```python
from build123d import *

# Parameters (mm, degrees)
SKETCH1_W           = 12.8
SKETCH1_H           = 5.8
BOSS_EXTRUDE1_DEPTH = 6.5
SKETCH2_R           = 1
CUT_EXTRUDE1_DEPTH  = 16.5
SKETCH3_W           = 0.9
SKETCH3_H           = 0.6
BOSS_EXTRUDE2_DEPTH = 3.5
BOSS_EXTRUDE3_DEPTH = 5.8
BOSS_EXTRUDE4_DEPTH = 2


with BuildPart() as part:
    # Sketch1 → Boss-Extrude1 (new body)
    with BuildSketch(Plane(origin=(0, 0, 0), x_dir=(1, 0, 0), z_dir=(0, 1, 0))):
        Rectangle(SKETCH1_W, SKETCH1_H)
    extrude(amount=BOSS_EXTRUDE1_DEPTH)

    # Sketch2 → Cut-Extrude1 (cut)
    with BuildSketch(Plane.XY.offset(2.9)):
        with Locations((-3.25, 1.4)):
            Circle(SKETCH2_R)
        with Locations((3.25, 1.4)):
            Circle(SKETCH2_R)
    extrude(amount=-CUT_EXTRUDE1_DEPTH, mode=Mode.SUBTRACT)

    # Sketch3 → Boss-Extrude2 (add)
    with BuildSketch(Plane.XZ):
        with Locations((-5.15, 0)):
            Rectangle(SKETCH3_W, SKETCH3_H)
        Rectangle(SKETCH3_W, SKETCH3_H)
        with Locations((5.15, 0)):
            Rectangle(SKETCH3_W, SKETCH3_H)
    extrude(amount=BOSS_EXTRUDE2_DEPTH)

    # Sketch4 → Boss-Extrude3 (add)
    with BuildSketch(Plane.XY.offset(2.9)):
        with BuildLine():
            Line((-3.1, 6.5), (-3.1, 7.3))
            ThreePointArc((-3.1, 7.3), (-2.1, 8.3), (-1.1, 7.3))
            Line((-1.1, 7.3), (-1.1, 6.5))
            Line((-1.1, 6.5), (-3.1, 6.5))
        make_face()
    extrude(amount=-BOSS_EXTRUDE3_DEPTH)

    # Sketch5 → Boss-Extrude4 (add, symmetric)
    with BuildSketch(Plane.XY):
        Polygon((-5.1, 6.5), (-5.1, 8.3), (8.241176471, 10.364705882), (8.294705882, 10.018823529), (-4.75, 8), (-4.75, 6.5), align=None)
    extrude(amount=BOSS_EXTRUDE4_DEPTH, both=True)


solid = part.part
```
Geometry: final body of the model. Coordinates: model frame, mm. A direction names the side the tool comes from. Give positions to 0.01 mm unless a question says otherwise; leave off trailing zeros. Order: outer loops, then holes, each group sorted by start corner. A loop starts at its lowest first (then second) coordinate and runs counter-clockwise, first axis right, second up. Notation, with made-up numbers: (32, 43) -> (76, 43) arc R12 cw to (76, 59) -> close; hole circle Ø2 at (21.5, -32). An arc over 180 degrees is marked (long way). Write each question's results on one line, items separated by ' | '. Start each with the question number.
1) Line query: line 1 (Y direction, x = -3.25, z = -0.05); line 2 (Y direction, x = 3.25, z = -0.85); line 3 (X direction, y = 0.75, z = 2.2). Output: solid intervals per line, ascending. Write a range as from..to.
2) Set-up query: faces 4 (the flat face through (5, -2, 0.3)), 5 (the flat face through (6.4, 3, 0)), 6 (the flat face through (0.6, 9, -2)), 7 (the flat face through (5, -2, -0.3)). Return all of +Z, -Z, +X, -X, +Y, -Y with unobstructed straight access to the full face (end or side cutting, diameter ignored); none if empty.
3) Draft query along X for faces 1 (the flat face through (0, -2, -0.3)), 2 (the cylindrical face through (-4.25, 1.44, 0.04)), 3 (the flat face through (-5.1, 7, 0)). Return one class per face: pulls with the +X half, pulls with the -X half, needs draft (parallel to the pull), parting line crosses it, or undercut.
4) Section C-C (x = 3.25). Return loops of the section in (y, z), then the cut area to 3 significant figures.
5) Section B-B (z = 1.05). Return loops of the section in (x, y).
6) First-contact query: pin 1 (3 mm diameter, centred on x = 2.5, z = -2, fed in from +Y); pin 2 (0.7 mm diameter, centred on x = 0, y = -2.5, fed in from -Z); pin 3 (0.9 mm diameter, centred on y = 7, z = 0, fed in from -X); pin 4 (1.6 mm diameter, centred on x = 3.25, y = 1.4, fed in from -Z). Flat tips, straight axial feed; report the tip coordinate or a pass-through.
7) Section D-D (y = 7.75). Return loops of the section in (x, z).
8) Section A-A (y = 1.4). Return loops of the section in (x, z), then the cut area to 3 significant figures.
Calculated:
1) line 1: 0..0.4, 2.4..6.5, 8.23..8.59 | line 2: 0..0.4, 2.4..6.5, 9.24..9.59 | line 3: -6.4..-4.01, -2.49..2.49, 4.01..6.4
2) face 4: +Z, +X, -X, -Y | face 5: +Z, -Z, +X, -Y | face 6: -Z, -X, +Y | face 7: -Z, +X, -X, -Y
3) face 1: needs draft | face 2: undercut | face 3: pulls with the -X half
4) outline: (0, -2.9) -> (0.4, -2.9) -> (0.4, 2.9) -> (0, 2.9) -> close; (2.4, -2.9) -> (6.5, -2.9) -> (6.5, 2.9) -> (2.4, 2.9) -> close; (9.24, -2) -> (9.59, -2) -> (9.59, 2) -> (9.24, 2) -> close | area: 27.5 mm2
5) outline: (-6.4, 0) -> (6.4, 0) -> (6.4, 6.5) -> (-1.1, 6.5) -> (-1.1, 7.3) arc R1 ccw to (-3.1, 7.3) -> (-3.1, 6.5) -> (-4.75, 6.5) -> (-4.75, 8) -> (8.29, 10.02) -> (8.24, 10.36) -> (-5.1, 8.3) -> (-5.1, 6.5) -> (-6.4, 6.5) -> close; hole circle Ø2 at (-3.25, 1.4); hole circle Ø2 at (3.25, 1.4)
6) pin 1: y = 9.71 | pin 2: z = -0.3 | pin 3: x = -5.1 | pin 4: through
7) outline: (-5.1, -2) -> (-4.75, -2) -> (-4.75, 2) -> (-5.1, 2) -> close; (-2.99, -2.9) -> (-1.21, -2.9) -> (-1.21, 2.9) -> (-2.99, 2.9) -> close
8) outline: (-6.4, -2.9) -> (-4.25, -2.9) -> (-4.25, 2.9) -> (-6.4, 2.9) -> close; (-2.25, -2.9) -> (2.25, -2.9) -> (2.25, 2.9) -> (-2.25, 2.9) -> close; (4.25, -2.9) -> (6.4, -2.9) -> (6.4, 2.9) -> (4.25, 2.9) -> close | area: 51.0 mm2
